from build123d import *

# Parameters (mm, degrees)
SKETCH_2_R          = 2.7
CUT_EXTRUDE_1_DEPTH = 10


with BuildPart() as part:
    # 草图1 → 旋转1 (revolve)
    with BuildSketch(Plane.XY, mode=Mode.PRIVATE) as revolve_1_sk:
        Polygon((0, 0), (0, 3.9), (9, 3.9), (9, 11), (63.9, 11), (63.9, 22), (66.3, 22), (66.3, 11), (66.3, 0), align=None)
    revolve(revolve_1_sk.sketch.rotate(Axis((0, 0, 0), (1, 0, 0)), 90), axis=Axis((0, 0, 0), (1, 0, 0)))

    # 草图2 → 切除-拉伸1 (cut)
    with BuildSketch(Plane.ZY.offset(-63.9)):
        with Locations((0, 17.5)):
            Circle(SKETCH_2_R)
        with Locations((15.155444566, -8.75)):
            Circle(SKETCH_2_R)
        with Locations((-15.155444566, -8.75)):
            Circle(SKETCH_2_R)
    extrude(amount=-CUT_EXTRUDE_1_DEPTH, mode=Mode.SUBTRACT)


solid = part.part
The listing builds one solid part. Answer for the finished solid, in the listing's coordinates (mm). A direction names the side the tool comes from. Round coordinates to 2 decimals unless told otherwise and drop trailing zeros. Write each loop counter-clockwise with the first axis right and the second up, starting at its lowest first coordinate (ties: lowest second). Pieces come first, ordered by that corner, then holes. Notation, with made-up numbers: M 44.25,-21 L 88.25,-21 A9 cw 88.25,-14 Z; hole C 2.5,4.25 d4. An arc over 180 degrees is marked long. Write each question's results on one line, items separated by ' | '. Start each with the question number.
Item 1: A cutting plane is placed at D-D on y = 0. Write down the section's boundary in (x, z), and give its area (3 significant figures).
Item 2: For faces 4 (the face through (0, 0, 0)), 5 (the face through (4.56, -2.64, -2.87)), determine the directions among +Z, -Z, +X, -X, +Y, -Y from which every point of the face is accessible in a straight line to the end or side of a thin tool.
Item 3: Straight lines are drawn through the part: L1, parallel to Y at x = 65.8, z = 0; L2, parallel to Z at x = 64, y = -8; L3, parallel to X at y = 4.5, z = -7.5. For each, find the intervals that lie inside material, in ascending order. Write a range as [from, to].
Item 4: A cutting plane is placed at A-A on z = 0. Write down the section's boundary in (x, y).
Item 5: A cutting plane is placed at C-C on y = 17.5. Write down the section's boundary in (x, z).
Item 6: A cutting plane is placed at B-B on y = -8.75. Write down the section's boundary in (x, z).
Item 7: Flat-ended cylindrical pins translate along their axes: pin 1 Ø2 at (x, z) = (10, 3) entering from +Y; pin 2 Ø6 at (y, z) = (-8.75, 15.16) entering from -X; pin 3 Ø1 at (x, y) = (58.5, 8) entering from +Z. Find the tip coordinate at first contact, or state that the pin passes through.
Item 8: For a pull along Z with two mould halves and no side action, classify faces 1 (the face through (65.117, 21.477, -4.769)), 2 (the face through (65.083, 20.177, -0.351)), 3 (the face through (66.3, 0, 0)) as pulls with the +Z half, pulls with the -Z half, needs draft (parallel to the pull), parting line crosses it, or undercut.
Check sheet entries:
1) outline: M 0,-3.9 L 9,-3.9 L 9,-11 L 63.9,-11 L 63.9,-22 L 66.3,-22 L 66.3,22 L 63.9,22 L 63.9,11 L 9,11 L 9,3.9 L 0,3.9 Z | area: 1,380 mm²
2) face 4: +Z, -Z, -X, +Y, -Y | face 5: -X
3) L1: [-22, 14.8], [20.2, 22] | L2: [-20.49, -17.75], [-12.56, 12.56], [17.75, 20.49] | L3: [9, 66.3]
4) outline: M 0,-3.9 L 9,-3.9 L 9,-11 L 63.9,-11 L 63.9,-22 L 66.3,-22 L 66.3,14.8 L 63.9,14.8 L 63.9,11 L 9,11 L 9,3.9 L 0,3.9 Z; M 63.9,20.2 L 66.3,20.2 L 66.3,22 L 63.9,22 Z
5) outline: M 63.9,-13.33 L 66.3,-13.33 L 66.3,-2.7 L 63.9,-2.7 Z; M 63.9,2.7 L 66.3,2.7 L 66.3,13.33 L 63.9,13.33 Z
6) outline: M 9,-6.67 L 63.9,-6.67 L 63.9,-12.46 L 66.3,-12.46 L 66.3,12.46 L 63.9,12.46 L 63.9,6.67 L 9,6.67 Z; M 63.9,-20.19 L 66.3,-20.19 L 66.3,-17.86 L 63.9,-17.86 Z; M 63.9,17.86 L 66.3,17.86 L 66.3,20.19 L 63.9,20.19 Z
7) pin 1: y = 10.82 | pin 2: x = 63.9 | pin 3: z = 8.05
8) face 1: parting line crosses it | face 2: undercut | face 3: needs draft
